```python
from build123d import *

# Parameters (mm, degrees)
F0_W     = 220.98
F0_H     = 120.65
F0_R     = 1.397
F1_DEPTH = 5.08
F2_W     = 214.63
F2_H     = 12.7
F2_R     = 1.397
F2_W_2   = 6.35
F2_H_2   = 95.25
F3_DEPTH = 5.08
F5_DEPTH = 25.4


# Not quite as in the source:
# - a feature names something its author has since deleted; it is built from what else it names


with BuildPart() as f1:
    # F0 (on Front) → F1 (new body)
    with BuildSketch(Plane.XZ):
        with Locations((110.49, 60.325)):
            Rectangle(F0_W, F0_H)
        with Locations((12.7, 6.35)):
            Circle(F0_R, mode=Mode.SUBTRACT)
        with Locations((208.28, 6.35)):
            Circle(F0_R, mode=Mode.SUBTRACT)
        with Locations((12.7, 114.3)):
            Circle(F0_R, mode=Mode.SUBTRACT)
        with Locations((208.28, 114.3)):
            Circle(F0_R, mode=Mode.SUBTRACT)
    extrude(amount=F1_DEPTH)

    # F2 (on face) → F3 (join)
    with BuildSketch(Plane.XZ.offset(5.08)):
        with Locations((113.665, 114.3)):
            Rectangle(F2_W, F2_H)
        with Locations((12.7, 114.3)):
            Circle(F2_R, mode=Mode.SUBTRACT)
        with Locations((208.28, 114.3)):
            Circle(F2_R, mode=Mode.SUBTRACT)
        with Locations((113.665, 6.35)):
            Rectangle(F2_W, F2_H)
        with Locations((12.7, 6.35)):
            Circle(F2_R, mode=Mode.SUBTRACT)
        with Locations((208.28, 6.35)):
            Circle(F2_R, mode=Mode.SUBTRACT)
        with Locations((3.175, 60.325)):
            Rectangle(F2_W_2, F2_H_2)
        with Locations((3.175, 114.3)):
            Rectangle(F2_W_2, F2_H)
        with Locations((3.175, 6.35)):
            Rectangle(F2_W_2, F2_H)
    extrude(amount=F3_DEPTH)

    # F4 (on face) → F5 (cut)
    with BuildSketch(Plane.XZ.offset(5.08)):
        with BuildLine():
            add(Edge.make_bspline(
                [(224.155, 85.725), (207.6572160579, 85.725), (215.906108029, 47.625), (224.155, 9.525), (232.403891971, 47.625), (240.6527839421, 85.725), (224.155, 85.725)],
                knots=[0, 0, 0, 2.0943951024, 2.0943951024, 4.1887902048, 4.1887902048, 6.2831853072, 6.2831853072, 6.2831853072], degree=2, weights=[1, 0.5, 1, 0.5, 1, 0.5, 1]))
        make_face()
    extrude(amount=-F5_DEPTH, mode=Mode.SUBTRACT)


solid = f1.part
```
Check sheet for the modelled part. Datum: model origin and axes. Units: mm. A direction names the side the tool comes from. Give positions to 0.01 mm unless a question says otherwise; leave off trailing zeros. Write each loop counter-clockwise with the first axis right and the second up, starting at its lowest first coordinate (ties: lowest second). Pieces come first, ordered by that corner, then holes. Notation, with made-up numbers: (36, 17.5) -> (75, 17.5) arc R10 ccw to (75, 34.5) -> close; hole circle Ø2 at (-35, -20.75). An arc over 180 degrees is marked (long way). Use CSV: the item, a comma, the result in double quotes. Start each with the question number.
Q1. Cross-section at A-A on y = -8. Enter the section's corners in (x, z).
Q2. Depth check by flat-ended pin: P1, Ø1, axis at y = -6, z = 49, coming from the +X side. Enter the tip coordinate at first touch or a pass-through.
Q3. Release check for a two-part mould opening along Z. For faces 1 (the flat face through (109, 0, 61)), 2 (the flat face through (109, -5, 0)), 3 (the flat face through (112, -8, 107.95)) record: +Z half, -Z half, draft (parallel to the pull), parting line (faces both ways), or undercut.
Q4. Cross-section at B-B on z = 87.5. Enter the section's corners in (x, y).
Q5. Cross-section at C-C on x = 84. Enter the section's corners in (y, z), and give its area (3 significant figures).
Q6. Tool access check on faces 4 (the flat face through (112, -8, 12.7)), 5 (the flat face through (0, -5, 61)). Record the directions out of +Z, -Z, +X, -X, +Y, -Y that give a thin tool (end or side, any length) a straight path to the whole face; none if there is none.
Q7. Scan lines: line 1 along Z through (x, y) = (12.7, -5.75); line 2 along Z through (x, y) = (208.28, -3.25); line 3 along Z through (x, y) = (123, -8.25). Record each from-to range of solid material in increasing order.
Working result:
1,outline,"(0, 0) -> (220.98, 0) -> (220.98, 12.7) -> (6.35, 12.7) -> (6.35, 107.95) -> (220.98, 107.95) -> (220.98, 120.65) -> (0, 120.65) -> close; hole circle Ø2.79 at (12.7, 6.35); hole circle Ø2.79 at (12.7, 114.3); hole circle Ø2.79 at (208.28, 6.35); hole circle Ø2.79 at (208.28, 114.3)"
2,P1,"stops at x = 6.35"
3,face 1,"draft"
3,face 2,"-Z half"
3,face 3,"undercut"
4,outline,"(0, -10.16) -> (6.35, -10.16) -> (6.35, -5.08) -> (220.98, -5.08) -> (220.98, 0) -> (0, 0) -> close"
5,outline,"(-10.16, 0) -> (0, 0) -> (0, 120.65) -> (-10.16, 120.65) -> (-10.16, 107.95) -> (-5.08, 107.95) -> (-5.08, 12.7) -> (-10.16, 12.7) -> close"
5,area,"742 mm^2"
6,face 4,"+X, -Y"
6,face 5,"+Z, -Z, -X, +Y, -Y"
7,line 1,"z = 0 to 4.95, 7.75 to 12.7, 107.95 to 112.9, 115.7 to 120.65"
7,line 2,"z = 0 to 4.95, 7.75 to 112.9, 115.7 to 120.65"
7,line 3,"z = 0 to 12.7, 107.95 to 120.65"
